```python
from build123d import *

# Parameters (mm, degrees)
ESTRUSIONE_ESTRUSIONE1_DEPTH = 120
FORO_FILETTATO_M3_1_D        = 2.5
FORO_FILETTATO_M3_1_DEPTH    = 10
FORO_FILETTATO_M3_1_TIP      = 0.751075774


with BuildPart() as part:
    # Schizzo1 → Estrusione-Estrusione1 (new body)
    with BuildSketch(Plane.XY):
        Polygon((0, 0), (-80, 0), (-80, -8), (-8, -8), (-8, -80), (0, -80), align=None)
    extrude(amount=ESTRUSIONE_ESTRUSIONE1_DEPTH)

    # Foro filettato M3-1
    with Locations(Plane.XY.offset(120)):
        with Locations((-10, -4), (-29, -4)):
            Hole(FORO_FILETTATO_M3_1_D / 2, depth=FORO_FILETTATO_M3_1_DEPTH)
            with Locations((0, 0, -(FORO_FILETTATO_M3_1_DEPTH + FORO_FILETTATO_M3_1_TIP / 2))):  # 118° drill point
                Cone(0, FORO_FILETTATO_M3_1_D / 2, FORO_FILETTATO_M3_1_TIP, mode=Mode.SUBTRACT)


solid = part.part
```
Can you work these out from the model? Positions are in its coordinate system, mm. A direction names the side the tool comes from. Round coordinates to 2 decimals unless told otherwise and drop trailing zeros. Loops run counter-clockwise (first coordinate to the right, second up) from the corner with the lowest first, then second, coordinate; pieces in that order, holes last. Notation, with made-up numbers: M -4,63 L 47,63 A12 cw 47,86 Z; hole C 10.25,-5 d4. An arc over 180 degrees is marked long. Write item = value, one per line. Start each with the question number.
(1) I'm going to push flat-ended pins straight in: P1, Ø10, axis at x = -43, z = 73.5, coming from the -Y side; P2, Ø6, axis at y = -66, z = 24.5, coming from the -X side; P3, Ø1.5, axis at y = -13.5, z = 86, coming from the +X side. Where does each tip first touch, or does it pass through?
(2) Suppose I cut it at B-B on y = -66.5. Write out the boundary of the cut face in (x, z), plus the area to 3 significant figures.
(3) I need wall thicknesses on line 1 along X through (y, z) = (-4, 114.25); line 2 along Y through (x, z) = (-10, 112); line 3 along Y through (x, z) = (-66, 77). Which ranges of each line are inside material? Lowest first, please.
(4) Which directions (+Z, -Z, +X, -X, +Y, -Y) give clear straight access to the entire face, cutting with the end or side of a thin tool? Please do faces 1 (the face through (-30.155, -4.479, 114.93)), 2 (the face through (-4, -80, 59)).
(5) If we mould it in two halves opening along Y, with no side actions, what happens to faces 3 (the face through (-9.01, -4.76, 114.93)), 4 (the face through (-45, -8, 59)), 5 (the face through (-8, -43, 59))? For each: released by +Y, released by -Y, zero draft, split by the parting line, or undercut.
(6) Suppose I cut it at A-A on z = 43. Write out the boundary of the cut face in (x, y).
Answer block:
q1.P1 = -8
q1.P2 = -8
q1.P3 = 0
q2.outline = M -8,0 L 0,0 L 0,120 L -8,120 Z
q2.area = 960 mm²
q3.line_1 = -80 to -30.25, -27.75 to -11.25, -8.75 to 0
q3.line_2 = -8 to -5.25, -2.75 to 0
q3.line_3 = -8 to 0
q4.face_1 = +Z
q4.face_2 = +Z, -Z, +X, -X, -Y
q5.face_3 = undercut
q5.face_4 = released by -Y
q5.face_5 = zero draft
q6.outline = M -80,-8 L -8,-8 L -8,-80 L 0,-80 L 0,0 L -80,0 Z
